Read the model definition and answer for the solid it produces. Units are mm, in the model's axes. Coordinates: 2 decimals unless noted, no trailing zeros. Loops run counter-clockwise (first coordinate to the right, second up) from the corner with the lowest first, then second, coordinate; pieces in that order, holes last.
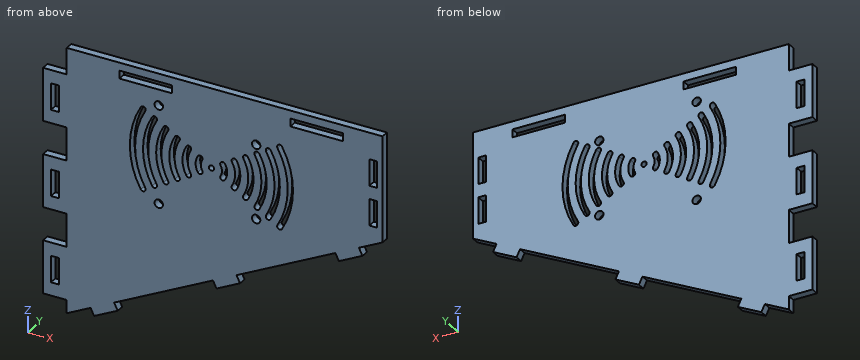
from build123d import *

# Parameters (mm, degrees)
SKETCH1_W           = 3
SKETCH1_H           = 10
SKETCH1_W_2         = 20
SKETCH1_H_2         = 3
BOSS_EXTRUDE1_DEPTH = 3
SKETCH2_R           = 1
SKETCH2_R_2         = 1.6
CUT_EXTRUDE1_DEPTH  = 3


with BuildPart() as part:
    # Sketch1 → Boss-Extrude1 (new body)
    with BuildSketch(Plane(origin=(0, 0, 0), x_dir=(1, 0, 0), z_dir=(0, 1, 0))):
        Polygon((0, 0), (0, 10), (-9, 10), (-9, 30), (0, 30), (0, 42.5), (-9, 42.5), (-9, 62.5), (0, 62.5), (0, 75), (-9, 75), (-9, 95), (0, 95), (0, 100), (9.091028316, 95.454485842), (10.432669103, 98.137767415), (19.376941013, 93.66563146), (18.035300226, 90.982349887), (55.601242248, 72.199378876), (56.942883035, 74.882660449), (65.887154945, 70.410524494), (64.545514158, 67.727242921), (102.11145618, 48.94427191), (103.453096967, 51.627553483), (112.397368877, 47.155417528), (111.05572809, 44.472135955), (120, 40), (120, 0), align=None)
        with Locations((116.5, 30)):
            Rectangle(SKETCH1_W, SKETCH1_H, mode=Mode.SUBTRACT)
        with Locations((116.5, 15)):
            Rectangle(SKETCH1_W, SKETCH1_H, mode=Mode.SUBTRACT)
        with Locations((30, 4.5)):
            Rectangle(SKETCH1_W_2, SKETCH1_H_2, mode=Mode.SUBTRACT)
        with Locations((95, 4.5)):
            Rectangle(SKETCH1_W_2, SKETCH1_H_2, mode=Mode.SUBTRACT)
        with Locations((-4.5, 85)):
            Rectangle(SKETCH1_W, SKETCH1_H, mode=Mode.SUBTRACT)
        with Locations((-4.5, 52.5)):
            Rectangle(SKETCH1_W, SKETCH1_H, mode=Mode.SUBTRACT)
        with Locations((-4.5, 20)):
            Rectangle(SKETCH1_W, SKETCH1_H, mode=Mode.SUBTRACT)
    extrude(amount=BOSS_EXTRUDE1_DEPTH)

    # Sketch2 → Cut-Extrude1 (cut)
    with BuildSketch(Plane.XZ):
        with Locations(Location((55, -30, 0), (0, 0, 270))):
            Circle(SKETCH2_R)
        with Locations(Location((35, -49, 0), (0, 0, 270))):
            Circle(SKETCH2_R_2)
        with Locations(Location((72, -44.5, 0), (0, 0, 270))):
            Circle(SKETCH2_R_2)
        with Locations(Location((72, -16.5, 0), (0, 0, 270))):
            Circle(SKETCH2_R_2)
        with Locations(Location((35, -12, 0), (0, 0, 270))):
            Circle(SKETCH2_R_2)
        with BuildLine():
            ThreePointArc((49.803847577, -27), (49, -30), (49.803847577, -33))
            ThreePointArc((49.803847577, -33), (51.169872981, -33.366025404), (51.535898385, -32))
            ThreePointArc((51.535898385, -32), (51, -30), (51.535898385, -28))
            ThreePointArc((51.535898385, -28), (51.169872981, -26.633974596), (49.803847577, -27))
        make_face()
        with BuildLine():
            ThreePointArc((45.473720558, -24.5), (44, -30), (45.473720558, -35.5))
            ThreePointArc((45.473720558, -35.5), (46.839745962, -35.866025404), (47.205771366, -34.5))
            ThreePointArc((47.205771366, -34.5), (46, -30), (47.205771366, -25.5))
            ThreePointArc((47.205771366, -25.5), (46.839745962, -24.133974596), (45.473720558, -24.5))
        make_face()
        with BuildLine():
            ThreePointArc((41.143593539, -22), (39, -30), (41.143593539, -38))
            ThreePointArc((41.143593539, -38), (42.509618943, -38.366025404), (42.875644347, -37))
            ThreePointArc((42.875644347, -37), (41, -30), (42.875644347, -23))
            ThreePointArc((42.875644347, -23), (42.509618943, -21.633974596), (41.143593539, -22))
        make_face()
        with BuildLine():
            ThreePointArc((36.813466521, -19.5), (34, -30), (36.813466521, -40.5))
            ThreePointArc((36.813466521, -40.5), (38.179491924, -40.866025404), (38.545517328, -39.5))
            ThreePointArc((38.545517328, -39.5), (36, -30), (38.545517328, -20.5))
            ThreePointArc((38.545517328, -20.5), (38.179491924, -19.133974596), (36.813466521, -19.5))
        make_face()
        with BuildLine():
            ThreePointArc((32.483339502, -17), (29, -30), (32.483339502, -43))
            ThreePointArc((32.483339502, -43), (33.849364905, -43.366025404), (34.215390309, -42))
            ThreePointArc((34.215390309, -42), (31, -30), (34.215390309, -18))
            ThreePointArc((34.215390309, -18), (33.849364905, -16.633974596), (32.483339502, -17))
        make_face()
        with BuildLine():
            ThreePointArc((28.153212483, -14.5), (24, -30), (28.153212483, -45.5))
            ThreePointArc((28.153212483, -45.5), (29.519237886, -45.866025404), (29.88526329, -44.5))
            ThreePointArc((29.88526329, -44.5), (26, -30), (29.88526329, -15.5))
            ThreePointArc((29.88526329, -15.5), (29.519237886, -14.133974596), (28.153212483, -14.5))
        make_face()
        with BuildLine():
            ThreePointArc((81.846787517, -14.5), (86, -30), (81.846787517, -45.5))
            ThreePointArc((81.846787517, -45.5), (80.480762114, -45.866025404), (80.11473671, -44.5))
            ThreePointArc((80.11473671, -44.5), (84, -30), (80.11473671, -15.5))
            ThreePointArc((80.11473671, -15.5), (80.480762114, -14.133974596), (81.846787517, -14.5))
        make_face()
        with BuildLine():
            ThreePointArc((77.516660498, -17), (81, -30), (77.516660498, -43))
            ThreePointArc((77.516660498, -43), (76.150635095, -43.366025404), (75.784609691, -42))
            ThreePointArc((75.784609691, -42), (79, -30), (75.784609691, -18))
            ThreePointArc((75.784609691, -18), (76.150635095, -16.633974596), (77.516660498, -17))
        make_face()
        with BuildLine():
            ThreePointArc((73.186533479, -19.5), (76, -30), (73.186533479, -40.5))
            ThreePointArc((73.186533479, -40.5), (71.820508076, -40.866025404), (71.454482672, -39.5))
            ThreePointArc((71.454482672, -39.5), (74, -30), (71.454482672, -20.5))
            ThreePointArc((71.454482672, -20.5), (71.820508076, -19.133974596), (73.186533479, -19.5))
        make_face()
        with BuildLine():
            ThreePointArc((68.856406461, -22), (71, -30), (68.856406461, -38))
            ThreePointArc((68.856406461, -38), (67.490381057, -38.366025404), (67.124355653, -37))
            ThreePointArc((67.124355653, -37), (69, -30), (67.124355653, -23))
            ThreePointArc((67.124355653, -23), (67.490381057, -21.633974596), (68.856406461, -22))
        make_face()
        with BuildLine():
            ThreePointArc((64.526279442, -24.5), (66, -30), (64.526279442, -35.5))
            ThreePointArc((64.526279442, -35.5), (63.160254038, -35.866025404), (62.794228634, -34.5))
            ThreePointArc((62.794228634, -34.5), (64, -30), (62.794228634, -25.5))
            ThreePointArc((62.794228634, -25.5), (63.160254038, -24.133974596), (64.526279442, -24.5))
        make_face()
        with BuildLine():
            ThreePointArc((60.196152423, -27), (61, -30), (60.196152423, -33))
            ThreePointArc((60.196152423, -33), (58.830127019, -33.366025404), (58.464101615, -32))
            ThreePointArc((58.464101615, -32), (59, -30), (58.464101615, -28))
            ThreePointArc((58.464101615, -28), (58.830127019, -26.633974596), (60.196152423, -27))
        make_face()
    extrude(amount=-CUT_EXTRUDE1_DEPTH, mode=Mode.SUBTRACT)


solid = part.part
Item 1: Given pin 1 (1 mm diameter, centred on x = 45, y = 2, fed in from -Z); pin 2 (0.9 mm diameter, centred on y = 1.5, z = -38, fed in from -X); pin 3 (1 mm diameter, centred on x = 60.5, y = 1, fed in from -Z), each flat-ended and moving along its own axis, determine where each tip first touches the part or whether it passes through.
Numbers:
pin 1: stops at z = -77.75
pin 2: stops at x = 0
pin 3: stops at z = -73.35
Item 2: A cutting plane is placed at A-A on z = -87. Determine the outline of the cut face in (x, y), then the cut area to 3 significant figures.
Numbers:
outline: (-9, 0) - (-6, 0) - (-6, 3) - (-9, 3) - close; (-3, 0) - (26, 0) - (26, 3) - (-3, 3) - close
area: 96.0 mm2
Item 3: Find the intervals of material crossed by line 1 along X through (y, z) = (0.8, -59.5); line 2 along X through (y, z) = (2.95, -50); line 3 along Z through (x, y) = (35.5, 2.75), in increasing order.
Numbers:
line 1: x = -9 to 81
line 2: x = -9 to -6, -3 to 33.75, 36.25 to 100, 102.64 to 106.71
line 3: z = -82.25 to -50.52, -47.48 to -37.79, -22.21 to -13.52, -10.48 to -6, -3 to 0
Item 4: A cutting plane is placed at B-B on y = 2. Give the number of separate pieces and of enclosed holes in the cut face, then the cut area to 3 significant figures.
Numbers:
separate pieces: 1
enclosed holes: 24
area: 8,250 mm2
